from build123d import *

# Parameters (mm, degrees)
BOSS_EXTRUDE1_DEPTH = 2.032
BOSS_EXTRUDE2_DEPTH = 17.78
CUT_EXTRUDE1_REACH  = 65.436
SKETCH4_R           = 3.429
CIRPATTERN1_COUNT   = 3
CIRPATTERN1_ANGLE   = 120


with BuildPart() as part:
    # Sketch1 → Boss-Extrude1 (new body)
    with BuildSketch(Plane(origin=(0, 0, 0), x_dir=(1, 0, 0), z_dir=(0, 1, 0))):
        Polygon((13.97, -24.196749782), (27.94, 0), (13.97, 24.196749782), (-13.97, 24.196749782), (-27.94, 0), (-13.97, -24.196749782), align=None)
        with BuildLine():
            Line((-9.0805, -1.4605), (-9.0805, 1.4605))
            Line((-9.0805, 1.4605), (-3.311754822, 1.4605))
            ThreePointArc((-3.311754822, 1.4605), (0.746285358, 3.541728168), (3.6195, 0))
            ThreePointArc((3.6195, 0), (0.746285358, -3.541728168), (-3.311754822, -1.4605))
            Line((-3.311754822, -1.4605), (-9.0805, -1.4605))
        make_face(mode=Mode.SUBTRACT)
    extrude(amount=BOSS_EXTRUDE1_DEPTH)

    # Sketch2 → Boss-Extrude2 (add)
    with BuildSketch(Plane.XZ):
        Polygon((13.97, 24.196749782), (-13.97, 24.196749782), (-27.94, 0), (-13.97, -24.196749782), (13.97, -24.196749782), (27.94, 0), align=None)
        Polygon((12.796824253, 22.164749782), (-12.796824253, 22.164749782), (-25.593648506, 0), (-12.796824253, -22.164749782), (12.796824253, -22.164749782), (25.593648506, 0), align=None, mode=Mode.SUBTRACT)
    extrude(amount=BOSS_EXTRUDE2_DEPTH)

    # Sketch4 → Cut-Extrude1 (cut, up to next)
    with BuildSketch(Plane(origin=(20.955, 0, -12.098374891), x_dir=(-0.49999999999999983, 0, -0.8660254037844387), z_dir=(0.8660254037844387, 0, -0.49999999999999983)), mode=Mode.PRIVATE) as cut_extrude1_sk1:
        with Locations((0, -6.477)):
            Circle(SKETCH4_R)
    cut_extrude1_tool1 = extrude(cut_extrude1_sk1.sketch, amount=-CUT_EXTRUDE1_REACH, mode=Mode.PRIVATE) & part.part
    cut_extrude1 = cut_extrude1_tool1.solids().sort_by_distance((20.955, -6.477, -12.098375))[0]
    add(cut_extrude1, mode=Mode.SUBTRACT)

    # CirPattern1: Cut-Extrude1 ×3 about axis
    cirpattern1_axis = Axis((0, 2.7686, 0), (0, 1, 0))
    for i in range(1, CIRPATTERN1_COUNT):
        add(cut_extrude1.rotate(cirpattern1_axis, i * CIRPATTERN1_ANGLE / (CIRPATTERN1_COUNT - 1)), mode=Mode.SUBTRACT)


solid = part.part
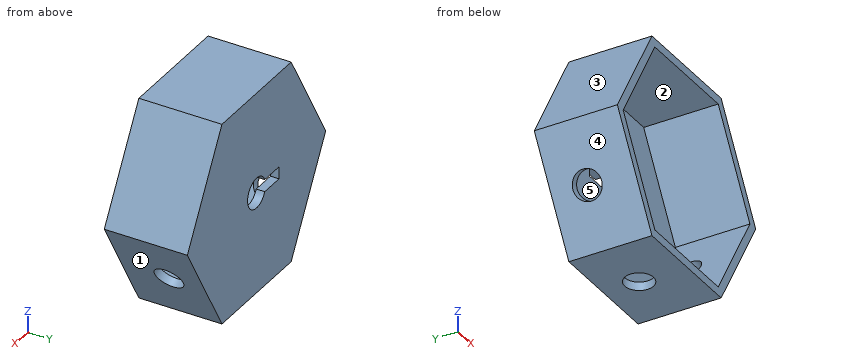
Verification items for the finished model (mm, model axes). Face numbers are marked on the shaded views. A direction names the side the tool comes from. Give positions to 0.01 mm unless a question says otherwise; leave off trailing zeros. Order: outer loops, then holes, each group sorted by start corner. A loop starts at its lowest first (then second) coordinate and runs counter-clockwise, first axis right, second up. Notation, with made-up numbers: M 60.5,-1 L 90.5,-1 A16 cw 90.5,9 Z; hole C 31.25,-6 d3. An arc over 180 degrees is marked long. Answer as a JSON object with one key per item and string values. Group by question number.
1) Scan lines: line 1 along Z through (x, y) = (-9, -7); line 2 along Z through (x, y) = (0, 1.25); line 3 along Y through (x, z) = (0, -23.3). Record each from-to range of solid material in increasing order. Write a range as [from, to].
2) Access from +Z, -Z, +X, -X, +Y, -Y to the whole of each face (thin tool, end or side, straight path). Record for the marked faces 4 and 5.
3) Cross-section at A-A (x = 0). Enter the section's corners in (y, z), then the cut area to 3 significant figures.
4) Cross-section at C-C (x = -12). Enter the section's corners in (y, z).
5) Depth check by flat-ended pin: pin 1 Ø3 at (x, z) = (-17, 9.5) entering from -Y; pin 2 Ø8 at (x, y) = (0, -6.477) entering from -Z; pin 3 Ø2 at (x, y) = (18.5, -11.5) entering from +Z; pin 4 Ø5 at (y, z) = (-6.5, 12) entering from +X. Enter the tip coordinate at first touch or a pass-through.
6) Cross-section at D-D (y = -9). Enter the section's corners in (x, z).
7) Mould release check, pull along Z, two halves, no side actions. Record for the marked faces 1, 2 and 3: released by +Z, released by -Z, zero draft, split by the parting line, or undercut.
8) Cross-section at B-B (y = -12.5). Enter the section's corners in (x, z).
Result sheet:
{
 "1": {"line 1": "z = [-24.2, -22.16], [22.16, 24.2]", "line 2": "z = [-24.2, -3.62], [3.62, 24.2]", "line 3": "y = [-17.78, -9.91], [-3.05, 2.03]"},
 "2": {"face 4": "-Z, -X, +Y, -Y", "face 5": "-Y"},
 "3": {"outline": "M -17.78,-24.2 L -9.91,-24.2 L -9.91,-22.16 L -17.78,-22.16 Z; M -17.78,22.16 L 0,22.16 L 0,3.62 L 2.03,3.62 L 2.03,24.2 L -17.78,24.2 Z; M -3.05,-24.2 L 2.03,-24.2 L 2.03,-3.62 L 0,-3.62 L 0,-22.16 L -3.05,-22.16 Z", "area": "142 mm2"},
 "4": {"outline": "M -17.78,-24.2 L 2.03,-24.2 L 2.03,24.2 L -17.78,24.2 L -17.78,22.16 L 0,22.16 L 0,-22.16 L -17.78,-22.16 Z"},
 "5": {"pin 1": "stops at y = 0", "pin 2": "stops at z = -24.2", "pin 3": "stops at z = 18.08", "pin 4": "stops at x = 22.46"},
 "6": {"outline": "M -27.94,0 L -22.12,-10.09 L -20.36,-9.07 L -25.59,0 L -12.8,22.16 L 12.8,22.16 L 25.59,0 L 20.36,-9.07 L 22.12,-10.09 L 27.94,0 L 13.97,24.2 L -13.97,24.2 Z; M -19.79,-14.11 L -13.97,-24.2 L -2.32,-24.2 L -2.32,-22.16 L -12.8,-22.16 L -18.03,-13.09 Z; M 2.32,-24.2 L 13.97,-24.2 L 19.79,-14.11 L 18.03,-13.09 L 12.8,-22.16 L 2.32,-22.16 Z"},
 "7": {"face 1": "released by -Z", "face 2": "undercut", "face 3": "released by +Z"},
 "8": {"outline": "M -27.94,0 L -13.97,-24.2 L 13.97,-24.2 L 27.94,0 L 13.97,24.2 L -13.97,24.2 Z; hole M -25.59,0 L -12.8,-22.16 L 12.8,-22.16 L 25.59,0 L 12.8,22.16 L -12.8,22.16 Z"}
}
